Design review of the part built by this model. Coordinates are the model's own, in mm. A direction names the side the tool comes from. Give positions to 0.01 mm unless a question says otherwise; leave off trailing zeros. Order: outer loops, then holes, each group sorted by start corner. A loop starts at its lowest first (then second) coordinate and runs counter-clockwise, first axis right, second up. Notation, with made-up numbers: M 50.25,68 L 54.25,68 A25 ccw 54.25,101 Z; hole C 34.5,23 d1. An arc over 180 degrees is marked long. Put each result on its own line as item: value. Start each with the question number.
from build123d import *

# Parameters (mm, degrees)
SKETCH_1_R          = 1.75
SKETCH_1_W          = 44
SKETCH_1_H          = 79
EXTRUDE_1_DEPTH     = 5
SKETCH_2_W          = 49
SKETCH_2_H          = 84
SKETCH_2_W_2        = 44
SKETCH_2_H_2        = 79
EXTRUDE_2_DEPTH     = 17
SKETCH_3_W          = 44.8
SKETCH_3_H          = 79.8
SKETCH_3_W_2        = 44
SKETCH_3_H_2        = 79
EXTRUDE_3_DEPTH     = 2
SKETCH_4_W          = 49
SKETCH_4_H          = 84
EXTRUDE_4_DEPTH     = 2
EXTRUDE_5_DEPTH     = 79
CUT_EXTRUDE_START   = 20
CUT_EXTRUDE_1_DEPTH = 10
SKETCH_7_R          = 1.75
CUT_EXTRUDE_2_DEPTH = 12.5
CUT_EXTRUDE_3_DEPTH = 91
SKETCH_9_R          = 3
SKETCH_9_R_2        = 1.75
EXTRUDE_6_DEPTH     = 10
SKETCH_11_W         = 6
SKETCH_11_H         = 10
SKETCH_11_R         = 1.75
EXTRUDE_7_DEPTH     = 3.5
CUT_EXTRUDE_4_DEPTH = 3.5
SKETCH_13_R         = 9.5
EXTRUDE_8_DEPTH     = 4
SKETCH_14_R         = 9.5
EXTRUDE_9_DEPTH     = 4
CUT_EXTRUDE_5_DEPTH = 2.5
SKETCH_16_R         = 1
CUT_EXTRUDE_6_DEPTH = 11
SKETCH_17_R         = 3.75
CUT_EXTRUDE_7_DEPTH = 3
SKETCH_18_R         = 1
CUT_EXTRUDE_8_DEPTH = 10.5


with BuildPart() as part:
    # Эскиз1 → Бобышка-Вытянуть1 (new body)
    with BuildSketch(Plane(origin=(0, 0, 0), x_dir=(1, 0, 0), z_dir=(0, 1, 0))):
        with BuildLine():
            Line((-3, -45), (-3, -44))
            ThreePointArc((-3, -44), (-3.585786438, -42.585786438), (-5, -42))
            Line((-5, -42), (-24.5, -42))
            Line((-24.5, -42), (-24.5, 42))
            Line((-24.5, 42), (-22.5, 42))
            ThreePointArc((-22.5, 42), (-21.085786438, 42.585786438), (-20.5, 44))
            Line((-20.5, 44), (-20.5, 45))
            ThreePointArc((-20.5, 45), (-17.5, 48), (-14.5, 45))
            Line((-14.5, 45), (-14.5, 44))
            ThreePointArc((-14.5, 44), (-13.914213562, 42.585786438), (-12.5, 42))
            Line((-12.5, 42), (12.5, 42))
            ThreePointArc((12.5, 42), (13.914213562, 42.585786438), (14.5, 44))
            Line((14.5, 44), (14.5, 45))
            ThreePointArc((14.5, 45), (17.5, 48), (20.5, 45))
            Line((20.5, 45), (20.5, 44))
            ThreePointArc((20.5, 44), (21.085786438, 42.585786438), (22.5, 42))
            Line((22.5, 42), (24.5, 42))
            Line((24.5, 42), (24.5, -42))
            Line((24.5, -42), (5, -42))
            ThreePointArc((5, -42), (3.585786438, -42.585786438), (3, -44))
            Line((3, -44), (3, -45))
            ThreePointArc((3, -45), (0, -48), (-3, -45))
        make_face()
        with Locations((-17.5, 45)):
            Circle(SKETCH_1_R, mode=Mode.SUBTRACT)
        with Locations((17.5, 45)):
            Circle(SKETCH_1_R, mode=Mode.SUBTRACT)
        with Locations((0, -45)):
            Circle(SKETCH_1_R, mode=Mode.SUBTRACT)
        Rectangle(SKETCH_1_W, SKETCH_1_H, mode=Mode.SUBTRACT)
    extrude(amount=EXTRUDE_1_DEPTH)

    # Эскиз2 → Бобышка-Вытянуть2 (add)
    with BuildSketch(Plane.XZ):
        Rectangle(SKETCH_2_W, SKETCH_2_H)
        Rectangle(SKETCH_2_W_2, SKETCH_2_H_2, mode=Mode.SUBTRACT)
    extrude(amount=EXTRUDE_2_DEPTH)

    # Эскиз3 → Бобышка-Вытянуть3 (add)
    with BuildSketch(Plane(origin=(0, 5, 0), x_dir=(1, 0, 0), z_dir=(0, 1, 0))):
        Rectangle(SKETCH_3_W, SKETCH_3_H)
        Rectangle(SKETCH_3_W_2, SKETCH_3_H_2, mode=Mode.SUBTRACT)
    extrude(amount=EXTRUDE_3_DEPTH)

    # Эскиз4 → Бобышка-Вытянуть4 (add)
    with BuildSketch(Plane.XZ.offset(17)):
        Rectangle(SKETCH_4_W, SKETCH_4_H)
    extrude(amount=EXTRUDE_4_DEPTH)

    # Эскиз5 → Бобышка-Вытянуть5 (add)
    with BuildSketch(Plane.XY.offset(-39.5)):
        with BuildLine():
            Line((3, -7.5), (-3, -7.5))
            ThreePointArc((-3, -7.5), (-5.782485579, -14.217514421), (-12.5, -17))
            Line((-12.5, -17), (12.5, -17))
            ThreePointArc((12.5, -17), (5.782485579, -14.217514421), (3, -7.5))
        make_face()
        with BuildLine():
            Line((-22, -17), (-12.5, -17))
            ThreePointArc((-12.5, -17), (-19.217514421, -14.217514421), (-22, -7.5))
            Line((-22, -7.5), (-22, -17))
        make_face()
        with BuildLine():
            ThreePointArc((22, -7.5), (19.217514421, -14.217514421), (12.5, -17))
            Line((12.5, -17), (22, -17))
            Line((22, -17), (22, -7.5))
        make_face()
    extrude(amount=EXTRUDE_5_DEPTH)

    # Эскиз6 → Вырез-Вытянуть1 (cut)
    with BuildSketch(Plane.XY.offset(-39.5).offset(CUT_EXTRUDE_START)):
        with BuildLine():
            Line((-2.042513515, -8.443915466), (2.042513515, -8.443915466))
            ThreePointArc((2.042513515, -8.443915466), (20.251164828, -14.583039164), (12.5, 3))
            Line((12.5, 3), (-12.5, 3))
            ThreePointArc((-12.5, 3), (-20.251164828, -14.583039164), (-2.042513515, -8.443915466))
        make_face()
    extrude(amount=CUT_EXTRUDE_1_DEPTH, mode=Mode.SUBTRACT)

    # Эскиз7 → Вырез-Вытянуть2 (cut, through all)
    with BuildSketch(Plane(origin=(0, -7.5, 0), x_dir=(1, 0, 0), z_dir=(0, 1, 0))):
        with Locations((0, 29.9)):
            Circle(SKETCH_7_R)
        with Locations((0, -29.9)):
            Circle(SKETCH_7_R)
    extrude(amount=-CUT_EXTRUDE_2_DEPTH, mode=Mode.SUBTRACT)

    # Эскиз8 → Вырез-Вытянуть3 (cut, through all)
    with BuildSketch(Plane.XY.offset(42)):
        with BuildLine():
            Line((-1.675248347, -9.5), (1.675248347, -9.5))
            ThreePointArc((1.675248347, -9.5), (3.339700343, -13.739279648), (6.519259302, -17))
            Line((6.519259302, -17), (6.519259302, -19))
            Line((6.519259302, -19), (-6.519259302, -19))
            Line((-6.519259302, -19), (-6.519259302, -17))
            ThreePointArc((-6.519259302, -17), (-3.339700343, -13.739279648), (-1.675248347, -9.5))
        make_face()
        with BuildLine():
            Line((19.480740698, -19), (24.5, -19))
            Line((24.5, -19), (24.5, -7.5))
            ThreePointArc((24.5, -7.5), (23.168050896, -12.872219372), (19.480740698, -17))
            Line((19.480740698, -17), (19.480740698, -19))
        make_face()
        with BuildLine():
            Line((-24.5, -7.5), (-24.5, -19))
            Line((-24.5, -19), (-19.480740698, -19))
            Line((-19.480740698, -19), (-19.480740698, -17))
            ThreePointArc((-19.480740698, -17), (-23.168050896, -12.872219372), (-24.5, -7.5))
        make_face()
    extrude(amount=-CUT_EXTRUDE_3_DEPTH, mode=Mode.SUBTRACT)

    # Эскиз9 → Бобышка-Вытянуть6 (add)
    with BuildSketch(Plane(origin=(0, -7.5, 0), x_dir=(1, 0, 0), z_dir=(0, 1, 0))):
        with Locations((0, 29.9)):
            Circle(SKETCH_9_R)
        with Locations((0, 29.9)):
            Circle(SKETCH_9_R_2, mode=Mode.SUBTRACT)
        with Locations((0, -29.9)):
            Circle(SKETCH_9_R)
        with Locations((0, -29.9)):
            Circle(SKETCH_9_R_2, mode=Mode.SUBTRACT)
    extrude(amount=EXTRUDE_6_DEPTH)

    # Эскиз11 → Бобышка-Вытянуть7 (add)
    with BuildSketch(Plane.XZ.offset(9.5)):
        with Locations((0, -29.9)):
            Rectangle(SKETCH_11_W, SKETCH_11_H)
        with Locations((0, -29.9)):
            Circle(SKETCH_11_R, mode=Mode.SUBTRACT)
        with Locations((0, 29.9)):
            Rectangle(SKETCH_11_W, SKETCH_11_H)
        with Locations((0, 29.9)):
            Circle(SKETCH_11_R, mode=Mode.SUBTRACT)
    extrude(amount=EXTRUDE_7_DEPTH)

    # Эскиз12 → Вырез-Вытянуть4 (cut)
    with BuildSketch(Plane.XZ.offset(13)):
        Polygon((0, 26.574462449), (2.88, 28.237231225), (2.88, 31.562768775), (0, 33.225537551), (-2.88, 31.562768775), (-2.88, 28.237231225), align=None)
        Polygon((0, -33.225537551), (2.88, -31.562768775), (2.88, -28.237231225), (0, -26.574462449), (-2.88, -28.237231225), (-2.88, -31.562768775), align=None)
    extrude(amount=-CUT_EXTRUDE_4_DEPTH, mode=Mode.SUBTRACT)

    # Эскиз13 → Бобышка-Вытянуть8 (add)
    with BuildSketch(Plane.XY.offset(-39.5)):
        with Locations((-12.5, -7.5)):
            Circle(SKETCH_13_R)
        with Locations((12.5, -7.5)):
            Circle(SKETCH_13_R)
    extrude(amount=EXTRUDE_8_DEPTH)

    # Эскиз14 → Бобышка-Вытянуть9 (add)
    with BuildSketch(Plane(origin=(0, 0, 39.5), x_dir=(-1, 0, 0), z_dir=(0, 0, -1))):
        with Locations((-12.5, -7.5)):
            Circle(SKETCH_14_R)
        with Locations((12.5, -7.5)):
            Circle(SKETCH_14_R)
    extrude(amount=EXTRUDE_9_DEPTH)

    # Эскиз15 → Вырез-Вытянуть5 (cut)
    with BuildSketch(Plane.XY.offset(-35.5)):
        Polygon((-12.5, -10.848631561), (-9.6, -9.174315781), (-9.6, -5.825684219), (-12.5, -4.151368439), (-15.4, -5.825684219), (-15.4, -9.174315781), align=None)
        Polygon((12.5, -10.848631561), (15.4, -9.174315781), (15.4, -5.825684219), (12.5, -4.151368439), (9.6, -5.825684219), (9.6, -9.174315781), align=None)
    extrude(amount=-CUT_EXTRUDE_5_DEPTH, mode=Mode.SUBTRACT)

    # Эскиз16 → Вырез-Вытянуть6 (cut, through all)
    with BuildSketch(Plane.XY.offset(-38)):
        with Locations((12.5, -7.5)):
            Circle(SKETCH_16_R)
        with Locations((-12.5, -7.5)):
            Circle(SKETCH_16_R)
    extrude(amount=-CUT_EXTRUDE_6_DEPTH, mode=Mode.SUBTRACT)

    # Эскиз17 → Вырез-Вытянуть7 (cut)
    with BuildSketch(Plane(origin=(0, 0, 35.5), x_dir=(-1, 0, 0), z_dir=(0, 0, -1))):
        with Locations((-12.5, -7.5)):
            Circle(SKETCH_17_R)
        with Locations((12.5, -7.5)):
            Circle(SKETCH_17_R)
    extrude(amount=-CUT_EXTRUDE_7_DEPTH, mode=Mode.SUBTRACT)

    # Эскиз18 → Вырез-Вытянуть8 (cut, through all)
    with BuildSketch(Plane(origin=(0, 0, 38.5), x_dir=(-1, 0, 0), z_dir=(0, 0, -1))):
        with Locations((-12.5, -7.5)):
            Circle(SKETCH_18_R)
        with Locations((12.5, -7.5)):
            Circle(SKETCH_18_R)
    extrude(amount=-CUT_EXTRUDE_8_DEPTH, mode=Mode.SUBTRACT)


solid = part.part
1. Machinability: for faces 1 (the cylindrical face through (3.31, -13.69, 0.59)), 2 (the cylindrical face through (-17.6, 2.5, -48)), 3 (the flat face through (22.4, 6, 1)), 4 (the flat face through (-14, -7, -38)), 5 (the flat face through (0, -7.5, -36)), which of the approach directions +Z, -Z, +X, -X, +Y, -Y give a long, thin tool a straight path to every point of the face, cutting with its end or side? Answer none if there is none.
2. To check wall thickness, follow probe 1 along Z at (x, y) = (0, -0.75); probe 2 along Z at (x, y) = (0, -8); probe 3 along Z at (x, y) = (-11.5, -16.75). State the ranges of each line that lie inside material, in increasing order.
3. The part is to be moulded in two halves that separate along X. For faces 6 (the flat face through (0, 0, 43)), 7 (the cylindrical face through (-0.65, -2.57, 32.83)), 8 (the cylindrical face through (3.6, 2.46, 42.57)), say which applies: +X half, -X half, draft (parallel to the pull), parting line (faces both ways), or undercut.
4. Consider section B-B on z = 21. Give the boundary of the cut face in (x, y), then the cut area to 3 significant figures.
5. Insertion check: pin 1 (15 mm diameter, centred on x = -13, y = -9, fed in from -Z); pin 2 (1.6 mm diameter, centred on x = -12.5, y = -7.5, fed in from -Z); pin 3 (6 mm diameter, centred on x = 11, y = -11.5, fed in from +Z); pin 4 (1.6 mm diameter, centred on y = -17.5, z = 7.5, fed in from +X). Each pin has a flat end and moves straight along its axis. Give the tip position at first contact, or say it passes through.
6. Consider section C-C on x = 7.5. Give the boundary of the cut face in (y, z), then the cut area to 3 significant figures.
7. Consider section A-A on x = -17.5. Give the boundary of the cut face in (y, z).
Returned:
1. face 1: -Y
1. face 2: -Z, +Y, -Y
1. face 3: +Z, -Z, +X, +Y
1. face 4: none
1. face 5: +Y
2. probe 1: z = -42 to -39.5, -32.9 to -31.65, -28.15 to -26.9, 26.9 to 28.15, 31.65 to 32.9, 39.5 to 42
2. probe 2: z = -42 to -31.65, -28.15 to -19.5, -9.5 to 28.15, 31.65 to 42
2. probe 3: z = -42 to -35.5, 35.5 to 42
3. face 6: draft
3. face 7: undercut
3. face 8: +X half
4. outline: M -24.5,-7.5 A11.5 ccw -19.48,-17 L -19.48,-19 L -6.52,-19 L -6.52,-17 A11.5 ccw -1.68,-9.5 L 1.68,-9.5 A11.5 ccw 6.52,-17 L 6.52,-19 L 19.48,-19 L 19.48,-17 A11.5 ccw 24.5,-7.5 L 24.5,5 L 22.4,5 L 22.4,7 L 22,7 L 22,-7.5 A9.5 cw 3,-7.5 L -3,-7.5 A9.5 cw -22,-7.5 L -22,7 L -22.4,7 L -22.4,5 L -24.5,5 Z
4. area: 219 mm2
5. pin 1: stops at z = -42
5. pin 2: passes through
5. pin 3: stops at z = 42
5. pin 4: stops at x = 19.9
6. outline: M -19,-42 L 5,-42 L 5,-39.9 L 7,-39.9 L 7,-39.5 L 0.58,-39.5 L 0.58,-35.5 L -15.58,-35.5 L -15.58,-19.5 L -16.73,-19.5 L -16.73,-9.5 L -15.58,-9.5 L -15.58,35.5 L 0.58,35.5 L 0.58,39.5 L 7,39.5 L 7,39.9 L 5,39.9 L 5,42 L -19,42 Z
6. area: 510 mm2
7. outline: M -19,-42 L 0,-42 L 0,-43.25 L 5,-43.25 L 5,-39.9 L 7,-39.9 L 7,-39.5 L 0.58,-39.5 L 0.58,-35.5 L -15.58,-35.5 L -15.58,-19.5 L -16.73,-19.5 L -16.73,-9.5 L -15.58,-9.5 L -15.58,35.5 L 0.58,35.5 L 0.58,39.5 L 7,39.5 L 7,39.9 L 5,39.9 L 5,42 L -19,42 Z; M 0,-48 L 5,-48 L 5,-46.75 L 0,-46.75 Z
